Part model, mm, in its own coordinate system. Coordinates: 2 decimals unless noted, no trailing zeros. Write each loop counter-clockwise with the first axis right and the second up, starting at its lowest first coordinate (ties: lowest second). Pieces come first, ordered by that corner, then holes. Notation, with made-up numbers: (-14.75, 48) - (12.25, 48) arc R10 ccw to (12.25, 52) - close; hole circle Ø10 at (4, 26.5). An arc over 180 degrees is marked (long way). Write each question's results on one line, items separated by ' | '.
Autodesk Inventor part; units mm, degrees
ref_plane "YZ Plane" through (0, 0, 0) normal (1, 0, 0) x (0, 1, 0)
ref_plane "XZ Plane" through (0, 0, 0) normal (0, 1, 0) x (-1, 0, 0)
ref_plane "XY Plane" through (0, 0, 0) normal (0, 0, 1) x (1, 0, 0)
sketch "Эскиз1" plane through (0, 0, 0) normal (0, 0, 1) x (1, 0, 0)
  line L0 (0, 0) -> (169.68, 0)
  line L1 (169.68, 0) -> (169.68, 60)
  line L2 (169.68, 60) -> (0, 60)
  line L3 (0, 60) -> (0, 0)
  dimension "d0" = 169.68
  dimension "d1" = 60
extrude "Выдавливание1" add sketch "Эскиз1" along normal blind 25
chamfer "Фаска1" distance 25 angle 45 2 edges at (0, 30, 25) (169.68, 30, 25)
sketch "Эскиз2" plane through (0, 60, 0) normal (0, 1, 0) x (1, 0, 0)
  line L0 (0, 0) -> (169.68, 0)
  line L1 (84.84, 0) -> (84.84, -96.7295)
  line L2 (169.68, 0) -> (0, 0)
  line L3 (25, -25) -> (144.68, -25)
  line L4 (0, 0) -> (25, -25)
  arc A0 (144.68, -25) -> (25, -25) centre (84.84, -285.0513) ccw
  line L5 (144.68, -25) -> (169.68, 0)
  arc A1 (159.68, -10) -> (10, -10) centre (84.84, -285.0513) ccw
  point P0 (169.68, -12)
  point P1 (0, -25)
  point P2 (169.68, -25)
  dimension "d7" = 10
extrude "Выдавливание2" cut sketch "Эскиз2" against normal blind 60 contours L0 A1 L4 | L0 L5 A1 | A0 L3 L1 | L1 L3 A0
properties part number "Long" material "Красное дерево"
(1) Saw through at B-B on x = 38.5. Write the cut outline in (y, z).
Return value:
outline: (0, 3.79) - (60, 3.79) - (60, 22.26) - (0, 22.26) - close
(2) Flat gauge pins, fed straight in: P1, Ø8, axis at x = 53, y = 50, coming from the +Z side; P2, Ø10, axis at x = 67.5, y = 29.5, coming from the -Z side; P3, Ø10, axis at x = 124, y = 54, coming from the -Z side; P4, Ø6, axis at x = 129, z = 12, coming from the -Y side. Where does each tip first touch, or does it go through?
Return value:
P1: stops at z = 20.62 | P2: stops at z = 0.27 | P3: stops at z = 2.05 | P4: stops at y = 0
(3) Two-plate mould, pull along X, no slides. Class faces 1 (the flat face through (84, 0, 12)), 2 (the flat face through (152.075, 30.42, 17.605)), 3 (the cylindrical face through (85.685, 30.42, 18.205)), 4 (the cylindrical face through (85.9, 30.4, 0)): released by +X, released by -X, zero draft, split by the parting line, or undercut.
Return value:
face 1: zero draft | face 2: released by +X | face 3: undercut | face 4: split by the parting line
(4) Saw through at C-C on y = 41.5. Write the cut outline in (x, z), then the cut area to 3 significant figures.
Return value:
outline: (10, 10) arc R285.05 ccw to (159.68, 10) - (144.68, 25) arc R266.85 cw to (25, 25) - close | area: 2,480 mm^2
(5) Saw through at A-A on z = 21. Write the cut outline in (x, y).
Return value:
outline: (21, 0) - (46.31, 0) - (46.31, 60) - (21, 60) - close; (123.37, 0) - (148.68, 0) - (148.68, 60) - (123.37, 60) - close
(6) Wall check: line 1 (Z direction, x = 87, y = 6); line 2 (Z direction, x = 58, y = 24); line 3 (X direction, y = 51, z = 10.5). Give the ranges that are in metal, low to high. Write a range as from..to.
Return value:
line 1: z = 0.01..18.21 | line 2: z = 1.27..19.56 | line 3: x = 10.5..159.18
